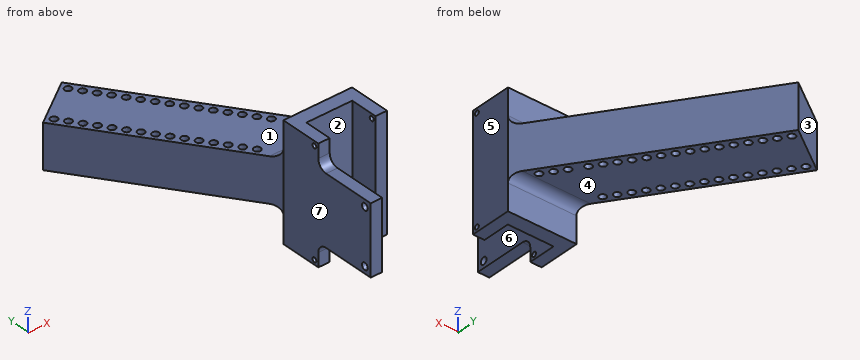
from build123d import *

# Parameters (mm, degrees)
BOSS_EXTRUDE1_DEPTH     = 50
SKETCH2_W               = 30
SKETCH2_H               = 27
SKETCH2_R               = 1.5
BOSS_EXTRUDE2_DEPTH     = 5
CUT_EXTRUDE1_DEPTH      = 65.257295306
CUT_EXTRUDE1_DEPTH_BACK = 65.257295306
SKETCH3_R               = 1
SKETCH5_W               = 19.2
SKETCH5_H               = 100
BOSS_EXTRUDE5_DEPTH     = 24.5
SKETCH5_2_W             = 19.2
SKETCH5_2_H             = 100
CUT_EXTRUDE3_DEPTH      = 80
SKETCH4_W               = 20
SKETCH4_H               = 21.42095117
CUT_EXTRUDE4_DEPTH      = 80
SKETCH9_R               = 1.5
CUT_EXTRUDE6_DEPTH      = 19.2
FILLET3_R               = 4
FILLET6_R               = 4


with BuildPart() as part:
    # Sketch1 → Boss-Extrude1 (new body)
    with BuildSketch(Plane.XY):
        Polygon((0, 0), (0, 18), (30, 18), (30, 0), (25, 0), (25, 12), (5, 12), (5, 0), align=None)
    extrude(amount=BOSS_EXTRUDE1_DEPTH)

    # Sketch2 → Boss-Extrude2 (add)
    with BuildSketch(Plane.ZY):
        with Locations((25, -13.5)):
            Rectangle(SKETCH2_W, SKETCH2_H)
        with Locations((13, -24)):
            Circle(SKETCH2_R, mode=Mode.SUBTRACT)
        with Locations(Location((37, -24, 0), (0, 0, 180))):
            Circle(SKETCH2_R, mode=Mode.SUBTRACT)
    extrude(amount=-BOSS_EXTRUDE2_DEPTH)

    # Sketch3 → Cut-Extrude1 (cut, two sides: drawn at the far end of the back side and taken through both)
    with BuildSketch(Plane(origin=(30, 0, 0), x_dir=(0, 0, -1), z_dir=(1, 0, 0)).offset(-CUT_EXTRUDE1_DEPTH_BACK)):
        with Locations(Location((-48, 2, 0), (0, 0, 90))):
            Circle(SKETCH3_R)
        with Locations(Location((-2, 2, 0), (0, 0, 180))):
            Circle(SKETCH3_R)
    extrude(amount=CUT_EXTRUDE1_DEPTH + CUT_EXTRUDE1_DEPTH_BACK, mode=Mode.SUBTRACT)

    # Sketch5 → Boss-Extrude5 (add, symmetric)
    with BuildSketch(Plane(origin=(28.587535737, 20.017208022, 0), x_dir=(0, 0, -1), z_dir=(0.8191520442889919, 0.573576436351046, 0))):
        with Locations((-25, 47.537443707)):
            Rectangle(SKETCH5_W, SKETCH5_H)
    extrude(amount=BOSS_EXTRUDE5_DEPTH, both=True)

    # Sketch5<2> → Cut-Extrude3 (cut)
    with BuildSketch(Plane(origin=(28.587535737, 20.017208022, 0), x_dir=(0, 0, -1), z_dir=(0.8191520442889919, 0.573576436351046, 0))):
        with Locations((-25, 47.537443707)):
            Rectangle(SKETCH5_2_W, SKETCH5_2_H)
    extrude(amount=CUT_EXTRUDE3_DEPTH, mode=Mode.SUBTRACT)

    # Sketch4 → Cut-Extrude4 (cut)
    with BuildSketch(Plane(origin=(0, 12, 0), x_dir=(1, 0, 0), z_dir=(0, 1, 0))):
        with Locations((15, -24.710475585)):
            Rectangle(SKETCH4_W, SKETCH4_H)
    extrude(amount=-CUT_EXTRUDE4_DEPTH, mode=Mode.SUBTRACT)

    # Sketch9 → Cut-Extrude6 (cut)
    with BuildSketch(Plane.XY.offset(34.6)):
        with Locations((-43.248683278, 85.125854914)):
            Circle(SKETCH9_R)
        with Locations((-40.380801097, 81.030094693)):
            Circle(SKETCH9_R)
        with Locations((-37.512918915, 76.934334472)):
            Circle(SKETCH9_R)
        with Locations((-34.645036733, 72.83857425)):
            Circle(SKETCH9_R)
        with Locations((-31.777154551, 68.742814029)):
            Circle(SKETCH9_R)
        with Locations((-28.909272369, 64.647053807)):
            Circle(SKETCH9_R)
        with Locations((-26.041390188, 60.551293586)):
            Circle(SKETCH9_R)
        with Locations((-23.173508006, 56.455533364)):
            Circle(SKETCH9_R)
        with Locations((-20.305625824, 52.359773143)):
            Circle(SKETCH9_R)
        with Locations((-17.437743642, 48.264012921)):
            Circle(SKETCH9_R)
        with Locations((-14.569861461, 44.1682527)):
            Circle(SKETCH9_R)
        with Locations((-11.701979279, 40.072492479)):
            Circle(SKETCH9_R)
        with Locations((-8.834097097, 35.976732257)):
            Circle(SKETCH9_R)
        with Locations((-5.966214915, 31.880972036)):
            Circle(SKETCH9_R)
        with Locations((-3.098332734, 27.785211814)):
            Circle(SKETCH9_R)
        with Locations((21.833754852, 24.432266344)):
            Circle(SKETCH9_R)
        with Locations((18.96587267, 28.528026566)):
            Circle(SKETCH9_R)
        with Locations((16.097990488, 32.623786787)):
            Circle(SKETCH9_R)
        with Locations((12.055980086, 38.396375887)):
            Circle(SKETCH9_R)
        with Locations((9.188097904, 42.492136108)):
            Circle(SKETCH9_R)
        with Locations((6.320215722, 46.58789633)):
            Circle(SKETCH9_R)
        with Locations((3.45233354, 50.683656551)):
            Circle(SKETCH9_R)
        with Locations((0.584451359, 54.779416773)):
            Circle(SKETCH9_R)
        with Locations((-2.283430823, 58.875176994)):
            Circle(SKETCH9_R)
        with Locations((-5.151313005, 62.970937215)):
            Circle(SKETCH9_R)
        with Locations((-8.019195187, 67.066697437)):
            Circle(SKETCH9_R)
        with Locations((-10.887077368, 71.162457658)):
            Circle(SKETCH9_R)
        with Locations((-13.75495955, 75.25821788)):
            Circle(SKETCH9_R)
        with Locations((-16.622841732, 79.353978101)):
            Circle(SKETCH9_R)
        with Locations((-19.490723914, 83.449738323)):
            Circle(SKETCH9_R)
        with Locations((-22.358606095, 87.545498544)):
            Circle(SKETCH9_R)
        with Locations((-25.226488277, 91.641258766)):
            Circle(SKETCH9_R)
        with Locations((-28.094370459, 95.737018987)):
            Circle(SKETCH9_R)
    extrude(amount=-CUT_EXTRUDE6_DEPTH, mode=Mode.SUBTRACT)

    # Fillet3
    fillet3_edges = [part.edges().sort_by_distance(p)[0] for p in [
        (15.045511288, 18, 34.6),
        (15.045511288, 18, 15.4),
    ]]
    fillet(fillet3_edges, radius=FILLET3_R)

    # Fillet6
    fillet6_edges = [part.edges().sort_by_distance(p)[0] for p in [
        (2.5, 0, 10),
        (2.5, 0, 40),
    ]]
    fillet(fillet6_edges, radius=FILLET6_R)


solid = part.part
Could you check a few things on this model? Use its own coordinates, in mm. Face numbers are marked on the shaded views. A direction names the side the tool comes from. Round coordinates to 2 decimals unless told otherwise and drop trailing zeros. Order: outer loops, then holes, each group sorted by start corner. A loop starts at its lowest first (then second) coordinate and runs counter-clockwise, first axis right, second up.
(1) Imagine slicing it at A-A (y = -24). Write out the boundary of the cut face in (x, z), plus the area to 3 significant figures.
Response values:
outline: (0, 10) - (5, 10) - (5, 11.5) - (0, 11.5) - close; (0, 14.5) - (5, 14.5) - (5, 35.5) - (0, 35.5) - close; (0, 38.5) - (5, 38.5) - (5, 40) - (0, 40) - close
area: 120 mm2
(2) Please list where these lines run through material, in increasing order: line 1 along Y through (x, z) = (28.85, 2); line 2 along X through (y, z) = (33, 23); line 3 along Y through (x, z) = (21.5, 45).
Response values:
line 1: y = 0 to 1, 3 to 18
line 2: x = -10.41 to -6.97, -4.97 to 14.65, 17.55 to 19.5
line 3: y = 12 to 18
(3) Imagine slicing it at C-C (z = 37). Write out the boundary of the cut face in (x, y), plus the area to 3 significant figures.
Response values:
outline: (-0.14, 18.33) - (0.09, 18) - (0, 18) - (0, -22.5) - (5, -22.5) - (5, 12) - (25, 12) - (25, 0) - (30, 0) - (30, 18) - (29.77, 18.33) - close; (0, -27) - (5, -27) - (5, -25.5) - (0, -25.5) - close
area: 430 mm2
(4) Which directions (+Z, -Z, +X, -X, +Y, -Y) give clear straight access to the entire face, cutting with the end or side of a thin tool? Please do the marked faces 1, 2, 3 and 4.
Response values:
face 1: +Z, +X, -X, +Y
face 2: +Z, -Z, -Y
face 3: +Z, -Z, -X, +Y
face 4: -Z, +X, -X, +Y
(5) Imagine slicing it at D-D (z = 29). Count the separate pieces of the cut face and the enclosed holes in it, plus the area to 3 significant figures.
Response values:
separate pieces: 1
enclosed holes: 33
area: 2,440 mm2
(6) If we mould it in two halves opening along X, with no side actions, what happens to the marked faces 5, 6 and 7? For each: released by +X, released by -X, zero draft, split by the parting line, or undercut.
Response values:
face 5: released by +X
face 6: undercut
face 7: released by -X
(7) I'm going to push flat-ended pins straight in: pin 1 (2.5 mm diameter, centred on x = 2.5, y = -15.5, fed in from +Z); pin 2 (4 mm diameter, centred on x = -8, y = 60.5, fed in from +Z); pin 3 (1.5 mm diameter, centred on x = 3.5, y = -20, fed in from -Z); pin 4 (12 mm diameter, centred on x = -27, z = 13.5, fed in from +Y). Where does each tip first touch, or does it pass through?
Response values:
pin 1: stops at z = 40
pin 2: stops at z = 34.6
pin 3: stops at z = 10
pin 4: stops at y = 99.92
(8) Imagine slicing it at B-B (x = 22). Write out the boundary of the cut face in (y, z), plus the area to 3 significant figures.
Response values:
outline: (12, 0) - (18, 0) - (18, 11.4) arc R4 cw to (22, 15.4) - (22.94, 15.4) - (22.94, 34.6) - (22, 34.6) arc R4 cw to (18, 38.6) - (18, 50) - (12, 50) - close; (25.92, 15.4) - (29.43, 15.4) - (29.43, 34.6) - (25.92, 34.6) - close
area: 469 mm2
